For this review, take the finished solid that the model builds, in its own axes (mm). Give positions to 0.01 mm unless a question says otherwise; leave off trailing zeros. Loops run counter-clockwise (first coordinate to the right, second up) from the corner with the lowest first, then second, coordinate; pieces in that order, holes last. Notation, with made-up numbers: M -20,41 L 25,41 A25 ccw 25,57 Z; hole C 11,-28 d4. An arc over 180 degrees is marked long. Use CSV: the item, a comma, the result in double quotes. Start each with the question number.
1. To check wall thickness, follow line 1 (Y direction, x = 11, z = 1.95) (3 decimals). State the ranges of the line that lie inside material, in increasing order. Write a range as [from, to].
2. Take a section at A-A, the plane x = 3. Write out the cut boundary in (y, z) (3 decimals).
3. Take a section at B-B, the plane z = 0.35. State how many separate pieces and enclosed holes the cut face has, and give its area (3 significant figures).
4. Insertion check: P1, Ø1.5, axis at x = 12.5, y = 2.5, coming from the -Z side. The pin has a flat end and moves straight along its axis. Give the tip position at first contact, or say it passes through.
from build123d import *

# Parameters (mm, degrees)
SKETCH1_W           = 22
SKETCH1_H           = 4.17
BOSS_EXTRUDE1_DEPTH = 4.47
SKETCH2_W           = 0.5
SKETCH2_H           = 0.5
CUT_EXTRUDE1_DEPTH  = 4.47


with BuildPart() as part:
    # Sketch1 → Boss-Extrude1 (new body)
    with BuildSketch(Plane.XY):
        with Locations((11, 2)):
            Rectangle(SKETCH1_W, SKETCH1_H)
    extrude(amount=BOSS_EXTRUDE1_DEPTH)

    # Sketch2 → Cut-Extrude1 (cut)
    with BuildSketch(Plane.XY.offset(4.47)):
        with Locations((1, 1)):
            Rectangle(SKETCH2_W, SKETCH2_H)
        with Locations((3, 1)):
            Rectangle(SKETCH2_W, SKETCH2_H)
        with Locations((5, 1)):
            Rectangle(SKETCH2_W, SKETCH2_H)
        with Locations((7, 1)):
            Rectangle(SKETCH2_W, SKETCH2_H)
        with Locations((9, 1)):
            Rectangle(SKETCH2_W, SKETCH2_H)
        with Locations((11, 1)):
            Rectangle(SKETCH2_W, SKETCH2_H)
        with Locations((13, 1)):
            Rectangle(SKETCH2_W, SKETCH2_H)
        with Locations((15, 1)):
            Rectangle(SKETCH2_W, SKETCH2_H)
        with Locations((17, 1)):
            Rectangle(SKETCH2_W, SKETCH2_H)
        with Locations((19, 1)):
            Rectangle(SKETCH2_W, SKETCH2_H)
        with Locations((21, 1)):
            Rectangle(SKETCH2_W, SKETCH2_H)
        with Locations((1, 3)):
            Rectangle(SKETCH2_W, SKETCH2_H)
        with Locations((3, 3)):
            Rectangle(SKETCH2_W, SKETCH2_H)
        with Locations((5, 3)):
            Rectangle(SKETCH2_W, SKETCH2_H)
        with Locations((7, 3)):
            Rectangle(SKETCH2_W, SKETCH2_H)
        with Locations((9, 3)):
            Rectangle(SKETCH2_W, SKETCH2_H)
        with Locations((11, 3)):
            Rectangle(SKETCH2_W, SKETCH2_H)
        with Locations((13, 3)):
            Rectangle(SKETCH2_W, SKETCH2_H)
        with Locations((15, 3)):
            Rectangle(SKETCH2_W, SKETCH2_H)
        with Locations((17, 3)):
            Rectangle(SKETCH2_W, SKETCH2_H)
        with Locations((19, 3)):
            Rectangle(SKETCH2_W, SKETCH2_H)
        with Locations((21, 3)):
            Rectangle(SKETCH2_W, SKETCH2_H)
    extrude(amount=-CUT_EXTRUDE1_DEPTH, mode=Mode.SUBTRACT)


solid = part.part
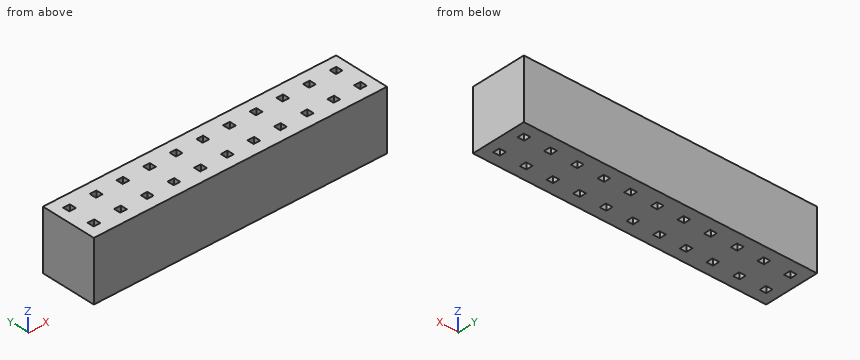
Result set:
1,line 1,"[-0.085, 0.75], [1.25, 2.75], [3.25, 4.085]"
2,outline,"M -0.085,0 L 0.75,0 L 0.75,4.47 L -0.085,4.47 Z; M 1.25,0 L 2.75,0 L 2.75,4.47 L 1.25,4.47 Z; M 3.25,0 L 4.085,0 L 4.085,4.47 L 3.25,4.47 Z"
3,separate pieces,"1"
3,enclosed holes,"22"
3,area,"86.2 mm2"
4,P1,"z = 0"
